```python
from build123d import *

# Parameters (mm, degrees)
F1_DEPTH = 9
F2_W     = 77.544987
F2_H     = 194.856629
F3_DEPTH = 9.001
F2_W_2   = 73.568299
F4_DEPTH = 9.001


with BuildPart() as f1:
    # F0 (on Top) → F1 (new body)
    with BuildSketch(Plane.XY):
        Polygon((143.506287, 346.454825), (-143.506287, 346.454825), (-346.454825, 143.506287), (-346.454825, -143.506287), (-143.506287, -346.454825), (143.506287, -346.454825), (346.454825, -143.506287), (346.454825, 143.506287), align=None)
    extrude(amount=F1_DEPTH)

    # F2 (on face) → F3 (cut, through all)
    with BuildSketch(Plane.XY):
        with Locations((277.869523, 22.715778)):
            Rectangle(F2_W, F2_H)
    extrude(amount=F3_DEPTH, mode=Mode.SUBTRACT)

    # F2 (on face) → F4 (cut, through all)
    with BuildSketch(Plane.XY):
        with Locations((-280.852013, 22.715778)):
            Rectangle(F2_W_2, F2_H)
    extrude(amount=F4_DEPTH, mode=Mode.SUBTRACT)


solid = f1.part
```
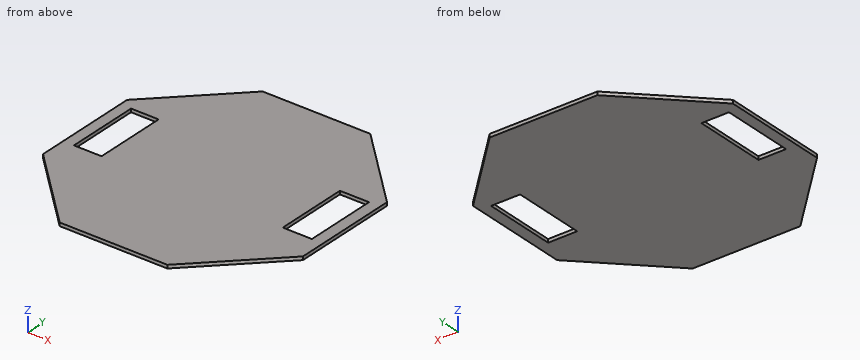
Can you work these out from the model? Positions are in its coordinate system, mm. Round coordinates to 2 decimals unless told otherwise and drop trailing zeros. Loops run counter-clockwise (first coordinate to the right, second up) from the corner with the lowest first, then second, coordinate; pieces in that order, holes last. Notation, with made-up numbers: M 18,27 L 54,27 A23 cw 54,50 Z; hole C 49.25,56.5 d9. An arc over 180 degrees is marked long. Answer as a JSON object with one key per item and string values. Group by question number.
Q1. Please list where these lines run through material, in increasing order: L1, parallel to X at y = -53.5, z = 1.25; L2, parallel to Y at x = -305, z = 5.75; L3, parallel to Y at x = -296, z = 3.
Q2. Imagine slicing it at D-D, the plane x = -296.5. Please give me the cut outline in (y, z), then the cut area to 3 significant figures.
Q3. Imagine slicing it at C-C, the plane x = 253. Please give me the cut outline in (y, z).
Q4. Imagine slicing it at B-B, the plane z = 5. Please give me the cut outline in (x, y).
Q5. Imagine slicing it at A-A, the plane y = -37.5. Please give me the cut outline in (x, z).
Q6. Will these pins go through, and if not, where does the flat tip stop? pin 1 (1.5 mm diameter, centred on y = 176.5, z = 1, fed in from -X); pin 2 (4.5 mm diameter, centred on x = 273, z = 4.5, fed in from -Y); pin 3 (3 mm diameter, centred on y = 261.5, z = 1, fed in from -X).
Findings:
{
 "1": {"L1": "x = -346.45 to -317.64, -244.07 to 239.1, 316.64 to 346.45", "L2": "y = -184.96 to -74.71, 120.14 to 184.96", "L3": "y = -193.96 to -74.71, 120.14 to 193.96"},
 "2": {"outline": "M -193.46,0 L -74.71,0 L -74.71,9 L -193.46,9 Z; M 120.14,0 L 193.46,0 L 193.46,9 L 120.14,9 Z", "area": "1,730 mm2"},
 "3": {"outline": "M -236.96,0 L -74.71,0 L -74.71,9 L -236.96,9 Z; M 120.14,0 L 236.96,0 L 236.96,9 L 120.14,9 Z"},
 "4": {"outline": "M -346.45,-143.51 L -143.51,-346.45 L 143.51,-346.45 L 346.45,-143.51 L 346.45,143.51 L 143.51,346.45 L -143.51,346.45 L -346.45,143.51 Z; hole M -317.64,-74.71 L -244.07,-74.71 L -244.07,120.14 L -317.64,120.14 Z; hole M 239.1,-74.71 L 316.64,-74.71 L 316.64,120.14 L 239.1,120.14 Z"},
 "5": {"outline": "M -346.45,0 L -317.64,0 L -317.64,9 L -346.45,9 Z; M -244.07,0 L 239.1,0 L 239.1,9 L -244.07,9 Z; M 316.64,0 L 346.45,0 L 346.45,9 L 316.64,9 Z"},
 "6": {"pin 1": "stops at x = -314.21", "pin 2": "stops at y = -219.21", "pin 3": "stops at x = -229.96"}
}
